For this review, take the finished solid that the model builds, in its own axes (mm). Coordinates: 2 decimals unless noted, no trailing zeros. Write each loop counter-clockwise with the first axis right and the second up, starting at its lowest first coordinate (ties: lowest second). Pieces come first, ordered by that corner, then holes.
```python
from build123d import *

# Parameters (mm, degrees)
F1_DEPTH = 14
F2_R     = 37.5
F3_DEPTH = 14


with BuildPart() as f1:
    # F0 (on Top) → F1 (new body)
    with BuildSketch(Plane.XY):
        Polygon((400, 0), (0, 0), (0, -50), (40, -50), (40, -150), (0, -150), (0, -200), (400, -200), (400, -150), (360, -150), (360, -50), (400, -50), align=None)
    extrude(amount=F1_DEPTH)

    # F2 (on face) → F3 (cut)
    with BuildSketch(Plane.XY.offset(14)):
        with Locations((195.744067, -100.478627)):
            Circle(F2_R)
    extrude(amount=-F3_DEPTH, mode=Mode.SUBTRACT)


solid = f1.part
```
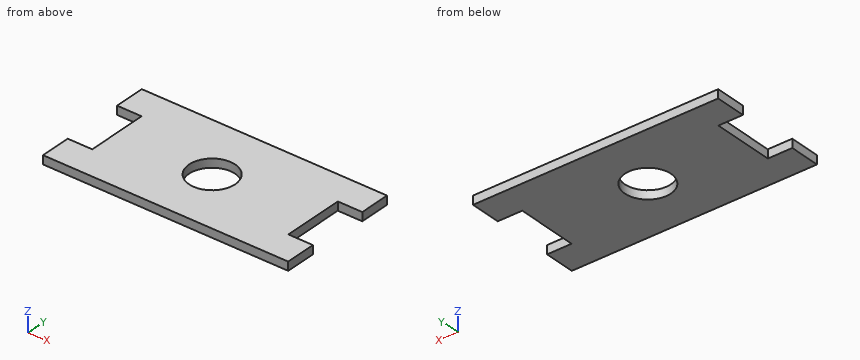
Q1. Add section B-B (x = 189.5). State the section outline as (y, z) points.
Ans:
outline: (-200, 0) - (-137.46, 0) - (-137.46, 14) - (-200, 14) - close; (-63.5, 0) - (0, 0) - (0, 14) - (-63.5, 14) - close
Q2. For probe 1 along Y at (x, z) = (28.5, 5.5); probe 2 along X at (y, z) = (-140.5, 7.75); probe 3 along X at (y, z) = (-89.5, 10), list the stretches that pass through material, from the lowest coordinate up.
Ans:
probe 1: y = -200 to -150, -50 to 0
probe 2: x = 40 to 360
probe 3: x = 40 to 159.89, 231.6 to 360
Q3. Add section C-C (z = 4.5). State the section outline as (x, y) points.
Ans:
outline: (0, -200) - (400, -200) - (400, -150) - (360, -150) - (360, -50) - (400, -50) - (400, 0) - (0, 0) - (0, -50) - (40, -50) - (40, -150) - (0, -150) - close; hole circle Ø75 at (195.74, -100.48)
Q4. Add section A-A (y = -120). State the section outline as (x, z) points, then the cut area to 3 significant figures.
Ans:
outline: (40, 0) - (163.73, 0) - (163.73, 14) - (40, 14) - close; (227.76, 0) - (360, 0) - (360, 14) - (227.76, 14) - close
area: 3,580 mm2
